```python
from build123d import *

# Parameters (mm, degrees)
SKETCH008_W     = 100
SKETCH008_H     = 11
PAD006_DEPTH    = 3
PAD007_DEPTH    = 5.35
SKETCH010_W     = 100
SKETCH010_H     = 11
PAD008_DEPTH    = 3
POCKET002_DEPTH = 5.35
FILLET005_R     = 1.23
FILLET006_R     = 1
SKETCH014_W     = 46.756413
SKETCH014_H     = 1.1
POCKET004_DEPTH = 12
FILLET007_R     = 1
SKETCH015_R     = 1.5
POCKET005_DEPTH = 2
SKETCH018_W     = 1
SKETCH018_H     = 6
PAD011_DEPTH    = 5.35


with BuildPart() as part:
    # Sketch008 → Pad006 (new body)
    with BuildSketch(Plane.XY):
        with Locations((-6.250698, -12.758651)):
            Rectangle(SKETCH008_W, SKETCH008_H)
    extrude(amount=PAD006_DEPTH)

    # Sketch009 (on Face6 of Pad006) → Pad007 (join)
    with BuildSketch(Plane.XY.offset(3)):
        Polygon((-56.250698, -13.258651), (33.992889, -13.258651), (33.992889, -9.258651), (43.492889, -13.258651), (46.749302, -13.258651), (46.749302, -15.758651), (58.749302, -15.758651), (58.749302, -18.258651), (-56.250698, -18.258651), align=None)
    extrude(amount=PAD007_DEPTH)

    # Sketch010 (on Face14 of Pad007) → Pad008 (join)
    with BuildSketch(Plane.XY.offset(8.35)):
        with Locations((-6.250698, -12.758651)):
            Rectangle(SKETCH010_W, SKETCH010_H)
    extrude(amount=PAD008_DEPTH)

    # Sketch011 (on Face14 of Pad007) → Pocket002 (cut)
    with BuildSketch(Plane.XY.offset(8.35)):
        Polygon((13.992889, -13.258651), (12.992889, -14.508651), (11.992889, -13.258651), align=None)
    extrude(amount=-POCKET002_DEPTH, mode=Mode.SUBTRACT)

    # Fillet005
    fillet005_edges = [part.edges().sort_by_distance(p)[0] for p in [
        (46.749302, -13.258651, 5.675),
        (46.749302, -15.758651, 5.675),
    ]]
    fillet(fillet005_edges, radius=FILLET005_R)

    # Fillet006
    fillet006_edges = [part.edges().sort_by_distance(p)[0] for p in [
        (58.749302, -15.758651, 5.675),
    ]]
    fillet(fillet006_edges, radius=FILLET006_R)

    # Sketch014 (on Face7 of Fillet006) → Pocket004 (cut)
    with BuildSketch(Plane.XZ.offset(18.258651)):
        with Locations((35.371096, 7.8)):
            Rectangle(SKETCH014_W, SKETCH014_H)
        with Locations((35.371096, 3.55)):
            Rectangle(SKETCH014_W, SKETCH014_H)
    extrude(amount=-POCKET004_DEPTH, mode=Mode.SUBTRACT)

    # Fillet007
    fillet007_edges = [part.edges().sort_by_distance(p)[0] for p in [
        (33.992889, -9.258651, 5.675),
    ]]
    fillet(fillet007_edges, radius=FILLET007_R)

    # Sketch015 (on Face34 of Fillet007) → Pocket005 (cut)
    with BuildSketch(Plane.XY.offset(11.35)):
        with Locations((-53.000698, -9.508651)):
            Circle(SKETCH015_R)
        with Locations((-49.750698, -12.758651)):
            Circle(SKETCH015_R)
        with Locations((-53.000698, -16.008651)):
            Circle(SKETCH015_R)
        with Locations((40.499302, -9.508651)):
            Circle(SKETCH015_R)
        with Locations((37.249302, -12.758651)):
            Circle(SKETCH015_R)
        with Locations((40.499302, -16.008651)):
            Circle(SKETCH015_R)
    pocket005 = extrude(amount=-POCKET005_DEPTH, mode=Mode.SUBTRACT)

    # Mirrored: Pocket005 across face of ReferencePlane
    add(pocket005.mirror(Plane(origin=(-57, -18, 5.5), x_dir=(1, 0, 0), z_dir=(0, 0, 1))), mode=Mode.SUBTRACT)

    # Sketch018 (on Face24 of Mirrored) → Pad011 (join)
    with BuildSketch(Plane.XY.offset(3)):
        with Locations((-55.750698, -10.258651)):
            Rectangle(SKETCH018_W, SKETCH018_H)
    extrude(amount=PAD011_DEPTH)


solid = part.part
```
For this review, take the finished solid that the model builds, in its own axes (mm). A direction names the side the tool comes from. Give positions to 0.01 mm unless a question says otherwise; leave off trailing zeros. Write each loop counter-clockwise with the first axis right and the second up, starting at its lowest first coordinate (ties: lowest second). Pieces come first, ordered by that corner, then holes. Notation, with made-up numbers: M 36,79 L 50,79 A23 ccw 50,102 Z; hole C 51,34.5 d4. An arc over 180 degrees is marked long. Answer as CSV lines item,"result".
1. Consider section A-A, the plane x = 28. Write out the cut boundary in (y, z).
Findings:
outline,"M -18.26,0 L -7.26,0 L -7.26,3 L -18.26,3 Z; M -18.26,4.1 L -13.26,4.1 L -13.26,7.25 L -18.26,7.25 Z; M -18.26,8.35 L -7.26,8.35 L -7.26,11.35 L -18.26,11.35 Z"
2. Draft analysis for pull direction X (two halves, no side actions). For faces 1 (the cylindrical face through (-54.19, -16.92, 0.81)), 2 (the flat face through (35, -16, 4.1)), 3 (the flat face through (40, -16, 1.65)), state which applies: +X half, -X half, draft (parallel to the pull), parting line (faces both ways), or undercut.
Findings:
face 1,"undercut"
face 2,"draft"
face 3,"undercut"
3. Consider section B-B, the plane x = -6.5. Write out the cut boundary in (y, z), then the cut area to 4 significant figures.
Findings:
outline,"M -18.26,0 L -7.26,0 L -7.26,3 L -13.26,3 L -13.26,8.35 L -7.26,8.35 L -7.26,11.35 L -18.26,11.35 Z"
area,"92.75 mm2"
4. Wall thickness on line 1 (X direction, y = -15.75, z = 0.75); line 2 (Z direction, x = 27.5, y = -10.5); line 3 (X direction, y = -11.5, z = 1.25): over which ranges is each line inside the solid? List them lowest first.
Findings:
line 1,"x = -56.25 to -54.48, -51.52 to 39.02, 41.98 to 43.75"
line 2,"z = 0 to 3, 8.35 to 11.35"
line 3,"x = -56.25 to -50.57, -48.93 to 36.43, 38.07 to 43.75"
5. For pin 1 (3.5 mm diameter, centred on x = -49, y = -12, fed in from -Z); pin 2 (3.5 mm diameter, centred on y = -11, z = 1, fed in from +X); pin 3 (2.5 mm diameter, centred on x = -25.5, z = 5.5, fed in from +Y); pin 4 (1.5 mm diameter, centred on x = -52.5, y = -10, fed in from +Z), all flat-tipped, find the tip position at first contact; note any pin that passes through.
Findings:
pin 1,"stops at z = 0"
pin 2,"stops at x = 43.75"
pin 3,"stops at y = -13.26"
pin 4,"stops at z = 9.35"
6. For faces 4 (the flat face through (-50, -13, 1.65)), 5 (the flat face through (53, -15.759, 6)), 6 (the flat face through (40, -9, 9.35)), 7 (the flat face through (-22, -13.259, 6)), list the 3-axis set-ups (+Z, -Z, +X, -X, +Y, -Y) from which the entire face can be reached by the end or side of a thin tool; tool diameter is ignored.
Findings:
face 4,"-Z"
face 5,"+Z, -Z, +X, +Y"
face 6,"+Z"
face 7,"+Y"
